Source: CAD feature listing. Evaluate the final solid. Frame: model axes, mm. Face numbers are marked on the shaded views. A direction names the side the tool comes from. Round coordinates to 2 decimals unless told otherwise and drop trailing zeros. Loops run counter-clockwise (first coordinate to the right, second up) from the corner with the lowest first, then second, coordinate; pieces in that order, holes last. Notation, with made-up numbers: (28, 45) - (81, 45) arc R7 cw to (81, 57) - close; hole circle Ø3 at (38, 33.25). An arc over 180 degrees is marked (long way). Use CSV: the item, a comma, the result in double quotes. Start each with the question number.
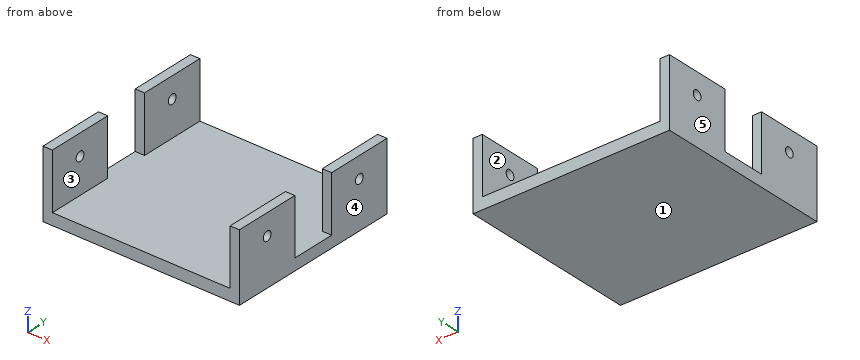
Autodesk Inventor part; units mm, degrees
ref_plane "YZ Plane" through (0, 0, 0) normal (1, 0, 0) x (0, 1, 0)
ref_plane "XZ Plane" through (0, 0, 0) normal (0, 1, 0) x (-1, 0, 0)
ref_plane "XY Plane" through (0, 0, 0) normal (0, 0, 1) x (1, 0, 0)
sketch "Эскиз1" plane through (0, 0, 0) normal (0, 0, 1) x (1, 0, 0)
  line L0 (-38, 52.38) -> (38, 52.38) construction
  line L1 (38, 52.38) -> (38, -52.38) construction
  line L2 (38, -52.38) -> (-38, -52.38) construction
  line L3 (-38, -52.38) -> (-38, 52.38) construction
  line L4 (-26.6205, -33.05) -> (26.6205, -33.05) construction
  line L5 (26.6205, -33.05) -> (26.6205, 33.05) construction
  line L6 (26.6205, 33.05) -> (-26.6205, 33.05) construction
  line L7 (-26.6205, 33.05) -> (-26.6205, -33.05) construction
  line L8 (0, 33.05) -> (0, 38.05) construction
  line L9 (0, -33.05) -> (0, -38.05) construction
  line L10 (-38, 38.05) -> (38, 38.05)
  line L11 (38, 38.05) -> (38, -38.05)
  line L12 (38, -38.05) -> (-38, -38.05)
  line L13 (-38, -38.05) -> (-38, 38.05)
  dimension "d0" = 76
  dimension "d1" = 104.76
  dimension "d2" = 53.241
  dimension "d3" = 66.1
  dimension "d4" = 5
  dimension "d5" = 5
extrude "Выдавливание1" add sketch "Эскиз1" along normal blind 5
sketch "Эскиз2" plane through (0, 0, 5) normal (0, 0, 1) x (1, 0, 0)
  line L0 (38, 38.05) -> (38, -38.05)
  line L1 (-38, -38.05) -> (-38, 38.05)
  line L2 (-38, 38.05) -> (-38, -38.05)
  line L3 (-38, -38.05) -> (-42, -38.05)
  line L4 (38, 38.05) -> (42, 38.05)
  line L5 (42, -38.05) -> (42, 38.05)
  line L6 (-42, 38.05) -> (-42, -38.05)
  line L7 (-38, -38.05) -> (-38, 38.05)
  line L8 (38, 38.05) -> (-38, 38.05)
  line L9 (38, 38.05) -> (38, -38.05)
  line L10 (42, 38.05) -> (38, 38.05)
  line L11 (-38, 38.05) -> (-42, 38.05)
  line L12 (-42, -38.05) -> (-38, -38.05)
  line L13 (38, -38.05) -> (42, -38.05)
  point P0 (0, 0)
  dimension "d8" = 4
  dimension "d9" = 4
extrude "Выдавливание2" add sketch "Эскиз2" along normal blind 24 and the other way blind 5
sketch "Эскиз3" plane through (0, 0, 29) normal (0, 0, 1) x (1, 0, 0)
  line L0 (38, 38.05) -> (38, -38.05)
  line L1 (38, -38.05) -> (42, -38.05)
  line L2 (42, -38.05) -> (42, 38.05)
  line L3 (42, 38.05) -> (38, 38.05)
  line L4 (42, 9.5) -> (38, 9.5)
  line L5 (38, 9.5) -> (38, -9.5)
  line L6 (38, -9.5) -> (42, -9.5)
  line L7 (42, -9.5) -> (42, 9.5)
  line L8 (42, 9.5) -> (38, -9.5) construction
  line L9 (38, 9.5) -> (42, -9.5) construction
  line L10 (0, 0) -> (0, -84) construction
  line L11 (-42, 9.5) -> (-38, 9.5)
  line L12 (-38, -9.5) -> (-42, -9.5)
  line L13 (-38, 9.5) -> (-38, -9.5) construction
  line L14 (-38, 38.05) -> (-38, -38.05) construction
  line L15 (-42, 9.5) -> (-42, -9.5) construction
  line L16 (-42, 38.05) -> (-42, -38.05) construction
  line L17 (-38, 9.5) -> (-38, -9.5)
  line L18 (-42, -9.5) -> (-42, 9.5)
  point P0 (40, 0)
  dimension "d14" = 4
  dimension "d15" = 19
extrude "Выдавливание3" cut sketch "Эскиз3" against normal up to surface (24 mm away) contours L4 L2 L6 L0 | L11 L17 L12 L18
sketch "Эскиз4" plane through (-42, 38.05, 0) normal (0, 1, 0) x (1, 0, 0)
  line L0 (0, 0) -> (84, 0)
  line L1 (0, 0) -> (0, -29)
  line L2 (4, -29) -> (0, -29)
  line L3 (4, -29) -> (4, -5)
  line L4 (80, -5) -> (4, -5)
  line L5 (80, -29) -> (80, -5)
  line L6 (84, -29) -> (80, -29)
  line L7 (84, 0) -> (84, -29)
  point P0 (42, 0)
sketch "Эскиз5" plane through (42, -38.05, 0) normal (1, 0, 0) x (0, 0, -1)
  line L0 (-29, 0) -> (-29, 28.55)
  line L1 (-29, 14.275) -> (-20, 14.275) construction
  circle A0 centre (-20, 14.275) radius 2
  line L2 (-5, 28.55) -> (-5, 47.55) construction
  line L3 (-5, 38.05) -> (-24.5, 38.05) construction
  circle A1 centre (-20, 61.825) radius 2
  point P0 (0, 38.05)
  dimension "d18" = 9
  dimension "d19" = 4
extrude "Выдавливание4" cut sketch "Эскиз5" against normal up to surface (84 mm away)
properties part number "Ard"
1. Section query B-B on z = 20. Give the number of separate pieces and of enclosed holes in the cut face, and give its area (3 significant figures).
2. Section query C-C on y = 32. Return the cut outline in (x, z).
3. Section query A-A on z = 6.75. Return the cut outline in (x, y).
4. Contact query for a flat-ended pin moving along its axis: P1, Ø2, axis at x = -24, y = -8.5, coming from the +Z side. Output: stop coordinate, or through.
5. Reachability of the marked faces 1 and 2 from +Z, -Z, +X, -X, +Y, -Y: full face, straight path, thin tool, end or side. Return the list, or none.
6. Mould query, pull axis X, two halves, no side actions, for the marked faces 3, 4 and 5. Classes: +X half, -X half, draft (parallel to the pull), parting line (faces both ways), or undercut.
7. Section query D-D on x = 14. Return the cut outline in (y, z).
8. Line query: line 1 along Y through (x, z) = (-40.3, 20) (3 decimals); line 2 along X through (y, z) = (33, 18); line 3 along Y through (x, z) = (38.5, 11.25). Output: solid intervals per line, ascending.
Values:
1,separate pieces,"8"
1,enclosed holes,"0"
1,area,"393 mm^2"
2,outline,"(-42, 0) - (42, 0) - (42, 29) - (38, 29) - (38, 5) - (-38, 5) - (-38, 29) - (-42, 29) - close"
3,outline,"(-42, -38.05) - (-38, -38.05) - (-38, -9.5) - (-42, -9.5) - close; (-42, 9.5) - (-38, 9.5) - (-38, 38.05) - (-42, 38.05) - close; (38, -38.05) - (42, -38.05) - (42, -9.5) - (38, -9.5) - close; (38, 9.5) - (42, 9.5) - (42, 38.05) - (38, 38.05) - close"
4,P1,"stops at z = 5"
5,face 1,"-Z, +X, -X, +Y, -Y"
5,face 2,"+Z, +Y, -Y"
6,face 3,"undercut"
6,face 4,"+X half"
6,face 5,"-X half"
7,outline,"(-38.05, 0) - (38.05, 0) - (38.05, 5) - (-38.05, 5) - close"
8,line 1,"y = -38.05 to -25.775, -21.775 to -9.5, 9.5 to 21.775, 25.775 to 38.05"
8,line 2,"x = -42 to -38, 38 to 42"
8,line 3,"y = -38.05 to -9.5, 9.5 to 38.05"
